Here's how the part is built. I have some questions about the finished solid (model axes, mm). A direction names the side the tool comes from. Round coordinates to 2 decimals unless told otherwise and drop trailing zeros. Order: outer loops, then holes, each group sorted by start corner. A loop starts at its lowest first (then second) coordinate and runs counter-clockwise, first axis right, second up. Notation, with made-up numbers: (70.25, 84.5) -> (111.25, 84.5) arc R14 cw to (111.25, 101.5) -> close; hole circle Ø2 at (43.5, 89). An arc over 180 degrees is marked (long way). Use a Markdown table: item, result. Add a question column.
(1) I want a section at B-B, the plane y = 58.5. Please give me the cut outline in (x, z), then the cut area to 3 significant figures.
(2) I want a section at D-D, the plane x = 0. Please give me the cut outline in (y, z), then the cut area to 3 significant figures.
(3) I want a section at C-C, the plane y = 84.5. Please give me the cut outline in (x, z), then the cut area to 3 significant figures.
(4) Thinking about a two-plate mould opening in X: for faces 6 (the face through (-48.47, 45.12, 86.35)), 7 (the face through (-1, 10, -27)), 8 (the face through (-54, 15, -16)), 9 (the face through (41.97, 4.93, 141.99)), which applies, pulls with the +X half, pulls with the -X half, needs draft (parallel to the pull), parting line crosses it, or undercut?
(5) On a 3-axis mill with a long thin cutter (end or side, diameter ignored), from which of +Z, -Z, +X, -X, +Y, -Y can I reach the whole of each face in a straight line? I mean faces 1 (the face through (48.47, 45.12, 86.35)), 2 (the face through (48.38, 55.93, -6.7)), 3 (the face through (-59.275, 19.345, -115.285)), 4 (the face through (54, 15, -16)), 5 (the face through (47.67, 44.51, 101.327)). Say none if no direction works.
(6) I want a section at A-A, the plane z = -65. Please give me the cut outline in (x, y), then the cut area to 3 significant figures.
(7) I'm going to push flat-ended pins straight in: P1, Ø1, axis at x = -20, z = -138.5, coming from the +Y side; P2, Ø16.5, axis at x = 49, z = -51, coming from the +Y side; P3, Ø8, axis at y = 36, z = -62.5, coming from the +X side; P4, Ø5, axis at x = -17.5, z = 31, coming from the -Y side. Where does each tip first touch, or does it pass through?
(8) If I drill on probe 1 along Y at (x, z) = (-34, -51); probe 2 along X at (y, z) = (12.5, 41); probe 3 along X at (y, z) = (28.5, 89.5), over which ranges is the centre line in solid material (lowest first)?
from build123d import *

# Parameters (mm, degrees)
EXTRUDE_1_DEPTH = 10
EXTRUDE_2_DEPTH = 10


with BuildPart() as part:
    # 草图1 → 凸台-拉伸1 (new body)
    with BuildSketch(Plane(origin=(0, 0, 0), x_dir=(1, 0, 0), z_dir=(0, 1, 0))):
        with BuildLine():
            Line((-65, 130), (-51.521169198, -121.604841641))
            ThreePointArc((-51.521169198, -121.604841641), (-42.202133258, -141.773208873), (-21.56412523, -150))
            Line((-21.56412523, -150), (21.56412523, -150))
            ThreePointArc((21.56412523, -150), (42.202133258, -141.773208873), (51.521169198, -121.604841641))
            Line((51.521169198, -121.604841641), (65, 130))
            ThreePointArc((65, 130), (0, 200), (-65, 130))
        make_face()
    extrude(amount=EXTRUDE_1_DEPTH)

    # 草图2 → 凸台-拉伸2 (add)
    with BuildSketch(Plane(origin=(57.86963434, 0, 3.100158983), x_dir=(0.053494721371611875, 0, -0.9985681322700888), z_dir=(0.9985681322700889, 0, 0.05349472137161188))):
        Polygon((-96.114027072, 89.677890258), (133.291014084, 30), (133.291014084, 10), (-98.63165297, 10), (-98.63165297, 80), align=None)
        Polygon((-83.63165297, 76.097869736), (118.291014084, 23.569299726), (118.291014084, 15), (-83.63165297, 15), align=None, mode=Mode.SUBTRACT)
    extrude_2 = extrude(amount=-EXTRUDE_2_DEPTH)

    # 镜向1: 凸台-拉伸2 across plane
    add(extrude_2.mirror(Plane(origin=(0, 0, 0), x_dir=(0, 0, 1), z_dir=(1, 0, 0))))


solid = part.part
Taken from the geometry:
| question | item | result |
|---|---|---|
| 1 | outline | (-59.14, -20.6) -> (-49.15, -21.14) -> (-47.03, 18.53) -> (-57.01, 19.06) -> close; (-53.4, 86.61) -> (-43.41, 86.08) -> (-42.61, 101.06) -> (-52.59, 101.59) -> close; (42.61, 101.06) -> (43.41, 86.08) -> (53.4, 86.61) -> (52.59, 101.59) -> close; (47.03, 18.53) -> (49.15, -21.14) -> (59.14, -20.6) -> (57.01, 19.06) -> close |
| 1 | area | 1,090 mm2 |
| 2 | outline | (0, -200) -> (10, -200) -> (10, 150) -> (0, 150) -> close |
| 2 | area | 3,500 mm2 |
| 3 | outline | (-53.79, 79.2) -> (-43.81, 78.67) -> (-42.67, 99.89) -> (-52.66, 100.42) -> close; (42.67, 99.89) -> (43.81, 78.67) -> (53.79, 79.2) -> (52.66, 100.42) -> close |
| 3 | area | 425 mm2 |
| 4 | face 6 | pulls with the -X half |
| 4 | face 7 | undercut |
| 4 | face 8 | needs draft |
| 4 | face 9 | pulls with the +X half |
| 5 | face 1 | +X |
| 5 | face 2 | -Z, +Y |
| 5 | face 3 | +Z |
| 5 | face 4 | +X, -X |
| 5 | face 5 | +Z, +Y |
| 6 | outline | (-61.52, 0) -> (61.52, 0) -> (61.52, 15) -> (51.5, 15) -> (51.5, 10) -> (-51.5, 10) -> (-51.5, 15) -> (-61.52, 15) -> close; (-61.52, 36.6) -> (-51.5, 36.74) -> (-51.5, 47.07) -> (-61.52, 46.93) -> close; (51.5, 36.74) -> (61.52, 36.6) -> (61.52, 46.93) -> (51.5, 47.07) -> close |
| 6 | area | 1,540 mm2 |
| 7 | P1 | stops at y = 10 |
| 7 | P2 | stops at y = 52.84 |
| 7 | P3 | stops at x = 61.6 |
| 7 | P4 | stops at y = 0 |
| 8 | probe 1 | y = 0 to 10 |
| 8 | probe 2 | x = -55.84 to -45.82, 45.82 to 55.84 |
| 8 | probe 3 | x = -53.24 to -43.23, 43.23 to 53.24 |
